from build123d import *

# Parameters (mm, degrees)
F0_W     = 7.62
F0_H     = 63.5
F1_DEPTH = 5.08
F4_D     = 7.239
F5_D     = 7.239


with BuildPart() as f1:
    # F0 (on Front) → F1 (new body)
    with BuildSketch(Plane.XZ):
        with Locations((-3.7611387034, 22.9711361981)):
            Rectangle(F0_W, F0_H)
    extrude(amount=F1_DEPTH)

    # F4 (through all)
    with Locations(Plane.XZ.offset(5.08)):
        with Locations((-3.7611387034, 48.3711361981)):
            Hole(F4_D / 2)

    # F5 (through all)
    with Locations(Plane(origin=(0, 0, 0), x_dir=(1, 0, 0), z_dir=(0, 1, 0))):
        with Locations((-3.7611387034, 2.4288638019)):
            Hole(F5_D / 2)


solid = f1.part
Work out the finished part from the listing and answer in its coordinate system (mm). Coordinates: 2 decimals unless noted, no trailing zeros. Write each loop counter-clockwise with the first axis right and the second up, starting at its lowest first coordinate (ties: lowest second). Pieces come first, ordered by that corner, then holes. Notation, with made-up numbers: M -2.75,-9.5 L 34.25,-9.5 A31 cw 34.25,20.5 Z; hole C -11,3 d7. An arc over 180 degrees is marked long. Use one line per item in the form item = value. Start each with the question number.
1. The part is cut by section A-A (x = -2.5). Give the vertices of the cut face in (y, z).
2. The part is cut by section C-C (x = -6.75). Give the vertices of the cut face in (y, z), plus the area to 3 significant figures.
3. The part is cut by section B-B (y = -2.3). Give the vertices of the cut face in (x, z).
4. The mould has two halves that part along Z. Classify faces 1 (the face through (-4, -3, 54.721)), 2 (the face through (-3.29, -2.5, 51.96)), 3 (the face through (0.049, -3, 23)): released by +Z, released by -Z, zero draft, split by the parting line, or undercut.
5. Straight lines are drawn through the part: probe 1 along Z at (x, y) = (-4, -1.35); probe 2 along Z at (x, y) = (-3, -0.3); probe 3 along X at (y, z) = (-3.1, 0.5). For each, find the intervals that lie inside material, in ascending order. Write a range as from..to.
Evaluation:
q1.outline = M -5.08,-8.78 L 0,-8.78 L 0,-5.82 L -5.08,-5.82 Z; M -5.08,0.96 L 0,0.96 L 0,44.98 L -5.08,44.98 Z; M -5.08,51.76 L 0,51.76 L 0,54.72 L -5.08,54.72 Z
q2.outline = M -5.08,-8.78 L 0,-8.78 L 0,-4.47 L -5.08,-4.47 Z; M -5.08,-0.39 L 0,-0.39 L 0,46.33 L -5.08,46.33 Z; M -5.08,50.41 L 0,50.41 L 0,54.72 L -5.08,54.72 Z
q2.area = 281 mm^2
q3.outline = M -7.57,-8.78 L 0.05,-8.78 L 0.05,54.72 L -7.57,54.72 Z; hole C -3.76,-2.43 d7.24; hole C -3.76,48.37 d7.24
q4.face_1 = released by +Z
q4.face_2 = undercut
q4.face_3 = zero draft
q5.probe_1 = -8.78..-6.04, 1.18..44.76, 51.98..54.72
q5.probe_2 = -8.78..-5.97, 1.11..44.83, 51.91..54.72
q5.probe_3 = -7.57..-5.89, -1.63..0.05
